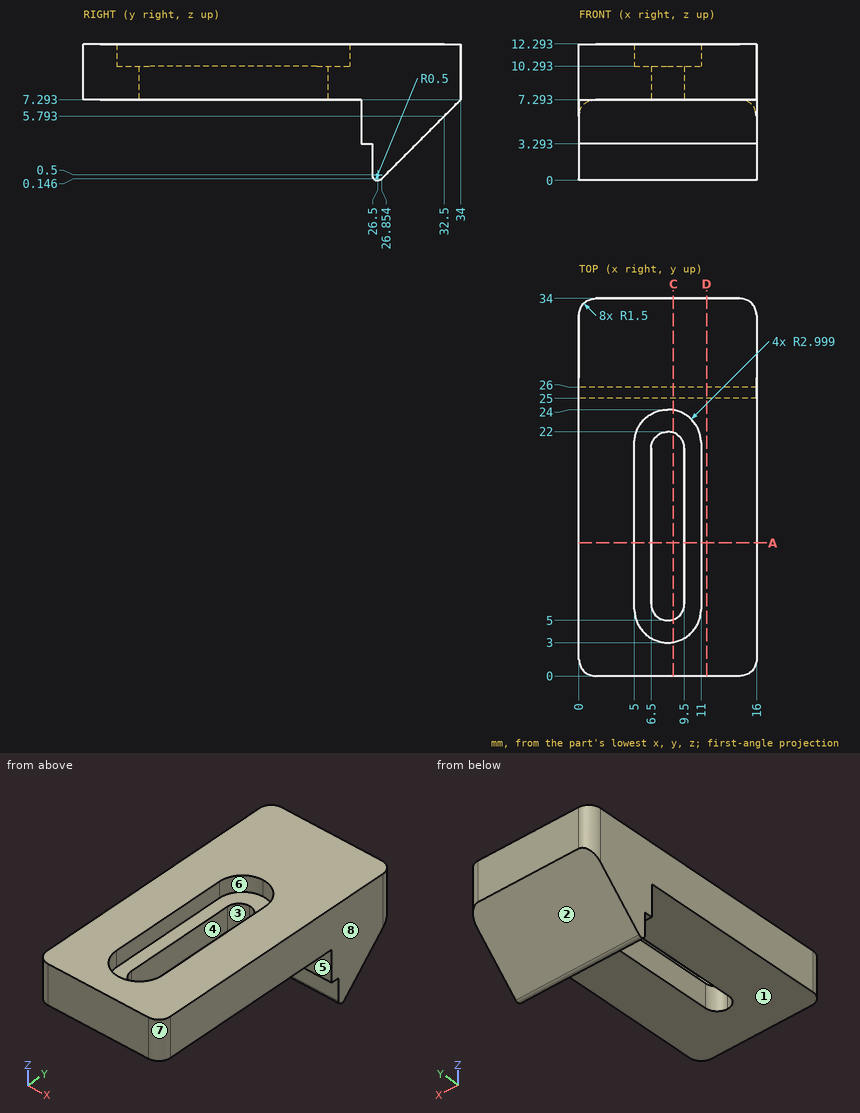
The drawing under review shows one solid part. Ordinate dimensions are in mm from its lowest x, y, z. A direction names the side the tool comes from. Round coordinates to 2 decimals unless told otherwise and drop trailing zeros. Loops run counter-clockwise (first coordinate to the right, second up) from the corner with the lowest first, then second, coordinate; pieces in that order, holes last. Notation, with made-up numbers: (47, 65.5) - (53, 65.5) arc R27 cw to (53, 98.5) - close; hole circle Ø6 at (44.5, 71.25). An arc over 180 degrees is marked (long way). One line per item, written item: value. Start each with the question number.
1) Insertion check: pin 1 Ø3 at (x, z) = (8, 5) entering from -Y; pin 2 Ø5 at (x, y) = (5.5, 7) entering from -Z; pin 3 Ø5 at (y, z) = (16.5, 2.5) entering from +X; pin 4 Ø1.4 at (x, z) = (5.5, 1.5) entering from -Y. Each pin has a flat end and moves straight along its axis. Give the tip position at first contact, or say it passes through.
2) Consider section D-D on x = 11.5. Give the boundary of the cut face in (y, z).
3) To check wall thickness, follow L1, parallel to X at y = 17.5, z = 10.5; L2, parallel to Z at x = 14.5, y = 15.5; L3, parallel to Z at x = 5.25, y = 7.5. State the ranges of each line that lie inside material, in increasing order. Write a range as from..to.
4) Draft analysis for pull direction Y (two halves, no side actions). For the marked faces 1, 2 and 3, state which applies: +Y half, -Y half, draft (parallel to the pull), parting line (faces both ways), or undercut.
5) Consider section A-A on y = 12. Give the boundary of the cut face in (x, z).
6) Consider section C-C on x = 8.5. Give the boundary of the cut face in (y, z) (1 decimal), then the cut area to 3 significant figures.
7) For the marked faces 4, 5, 6, 7 and 8, list the 3-axis set-ups (+Z, -Z, +X, -X, +Y, -Y) from which the entire face can be reached by the end or side of a thin tool; tool diameter is ignored.
Reported:
1. pin 1: stops at y = 25
1. pin 2: stops at z = 7.29
1. pin 3: passes through
1. pin 4: stops at y = 26
2. outline: (0, 7.29) - (25, 7.29) - (25, 3.29) - (26, 3.29) - (26, 0.5) arc R0.5 ccw to (26.85, 0.15) - (34, 7.29) - (34, 12.29) - (0, 12.29) - close
3. L1: x = 0..5, 11..16
3. L2: z = 7.29..12.29
3. L3: z = 7.29..10.29
4. face 1: draft
4. face 2: +Y half
4. face 3: undercut
5. outline: (0, 7.29) - (6.5, 7.29) - (6.5, 10.29) - (5, 10.29) - (5, 12.29) - (0, 12.29) - close; (9.5, 7.29) - (16, 7.29) - (16, 12.29) - (11, 12.29) - (11, 10.29) - (9.5, 10.29) - close
6. outline: (0, 7.3) - (5.1, 7.3) - (5.1, 10.3) - (3, 10.3) - (3, 12.3) - (0, 12.3) - close; (21.9, 7.3) - (25, 7.3) - (25, 3.3) - (26, 3.3) - (26, 0.5) arc R0.5 ccw to (26.9, 0.1) - (34, 7.3) - (34, 12.3) - (24, 12.3) - (24, 10.3) - (21.9, 10.3) - close
6. area: 113 mm^2
7. face 4: +Z, -Z
7. face 5: -Z, +X, -X, -Y
7. face 6: +Z
7. face 7: +Z, -Z, +X, -Y
7. face 8: +Z, -Z, +X, +Y, -Y
